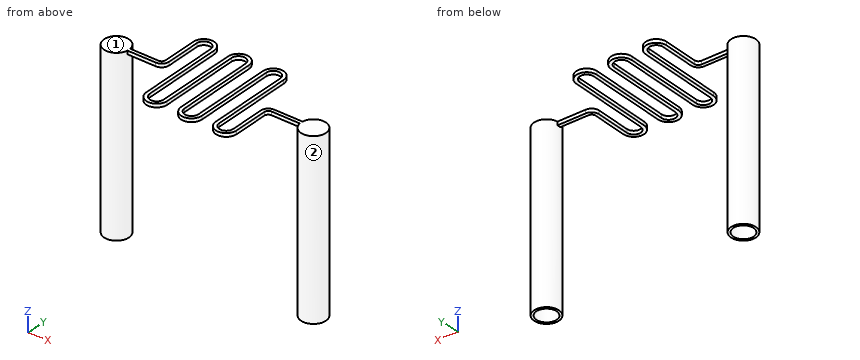
from build123d import *

# Parameters (mm, degrees)
BOSS_EXTRUDE1_DEPTH = 0.6
SKETCH3_W           = 2.15
SKETCH3_H           = 30
SKETCH4_W           = 2.15
SKETCH4_H           = 30
SKETCH5_R           = 1.75
CUT_EXTRUDE1_DEPTH  = 29


with BuildPart() as part:
    # Sketch2 → Boss-Extrude1 (new body)
    with BuildSketch(Plane.XY):
        with BuildLine():
            Line((-20.5, -0.3), (-13.5, -0.3))
            ThreePointArc((-13.5, -0.3), (-12.580761184, 0.080761184), (-12.2, 1))
            Line((-12.2, 1), (-12.2, 7))
            ThreePointArc((-12.2, 7), (-11, 8.2), (-9.8, 7))
            Line((-9.8, 7), (-9.8, 0))
            Line((-9.8, 0), (-9.8, -7))
            ThreePointArc((-9.8, -7), (-8, -8.8), (-6.2, -7))
            Line((-6.2, -7), (-6.2, 0))
            Line((-6.2, 0), (-6.2, 7))
            ThreePointArc((-6.2, 7), (-5, 8.2), (-3.8, 7))
            Line((-3.8, 7), (-3.8, 0))
            Line((-3.8, 0), (-3.8, -7))
            ThreePointArc((-3.8, -7), (-2, -8.8), (-0.2, -7))
            Line((-0.2, -7), (-0.2, 0))
            Line((-0.2, 0), (-0.2, 7))
            ThreePointArc((-0.2, 7), (1, 8.2), (2.2, 7))
            Line((2.2, 7), (2.2, 0))
            Line((2.2, 0), (2.2, -7))
            ThreePointArc((2.2, -7), (4, -8.8), (5.8, -7))
            Line((5.8, -7), (5.8, -1))
            ThreePointArc((5.8, -1), (6.005025253, -0.505025253), (6.5, -0.3))
            Line((6.5, -0.3), (13.5, -0.3))
            ThreePointArc((13.5, -0.3), (13.8, 0), (13.5, 0.3))
            Line((13.5, 0.3), (6.5, 0.3))
            ThreePointArc((6.5, 0.3), (5.580761184, -0.080761184), (5.2, -1))
            Line((5.2, -1), (5.2, -7))
            ThreePointArc((5.2, -7), (4, -8.2), (2.8, -7))
            Line((2.8, -7), (2.8, 0))
            Line((2.8, 0), (2.8, 7))
            ThreePointArc((2.8, 7), (1, 8.8), (-0.8, 7))
            Line((-0.8, 7), (-0.8, 0))
            Line((-0.8, 0), (-0.8, -7))
            ThreePointArc((-0.8, -7), (-2, -8.2), (-3.2, -7))
            Line((-3.2, -7), (-3.2, 0))
            Line((-3.2, 0), (-3.2, 7))
            ThreePointArc((-3.2, 7), (-5, 8.8), (-6.8, 7))
            Line((-6.8, 7), (-6.8, 0))
            Line((-6.8, 0), (-6.8, -7))
            ThreePointArc((-6.8, -7), (-8, -8.2), (-9.2, -7))
            Line((-9.2, -7), (-9.2, 0))
            Line((-9.2, 0), (-9.2, 7))
            ThreePointArc((-9.2, 7), (-11, 8.8), (-12.8, 7))
            Line((-12.8, 7), (-12.8, 1))
            ThreePointArc((-12.8, 1), (-13.005025253, 0.505025253), (-13.5, 0.3))
            Line((-13.5, 0.3), (-20.5, 0.3))
            ThreePointArc((-20.5, 0.3), (-20.8, 0), (-20.5, -0.3))
        make_face()
    extrude(amount=BOSS_EXTRUDE1_DEPTH)

    # Sketch3 → Revolve1 (revolve)
    with BuildSketch(Plane(origin=(0, 0, 0), x_dir=(1, 0, 0), z_dir=(0, 1, 0))):
        with Locations((-21.575, 14.4)):
            Rectangle(SKETCH3_W, SKETCH3_H)
    revolve(axis=Axis((-20.5, 0, -29.4), (0, 0, 1)))

    # Sketch4 → Revolve2 (revolve)
    with BuildSketch(Plane(origin=(0, 0, 0), x_dir=(1, 0, 0), z_dir=(0, 1, 0)), mode=Mode.PRIVATE) as revolve2_sk:
        with Locations((14.575, 14.4)):
            Rectangle(SKETCH4_W, SKETCH4_H)
    revolve(revolve2_sk.sketch.rotate(Axis((13.5, 0, -29.4), (0, 0, 1)), 180), axis=Axis((13.5, 0, -29.4), (0, 0, 1)))

    # Sketch5 → Cut-Extrude1 (cut)
    with BuildSketch(Plane(origin=(0, 0, -29.4), x_dir=(-1, 0, 0), z_dir=(0, 0, -1))):
        with Locations((20.5, 0)):
            Circle(SKETCH5_R)
        with Locations((-13.5, 0)):
            Circle(SKETCH5_R)
    extrude(amount=-CUT_EXTRUDE1_DEPTH, mode=Mode.SUBTRACT)


solid = part.part
Input: part model. Units: mm. Frame: model coordinates. Face numbers are marked on the shaded views. Give positions to 0.01 mm unless a question says otherwise; leave off trailing zeros. Loops run counter-clockwise (first coordinate to the right, second up) from the corner with the lowest first, then second, coordinate; pieces in that order, holes last. Notation, with made-up numbers: (43, 32.25) -> (85, 32.25) arc R28 cw to (85, 61.25) -> close; hole circle Ø3 at (4.5, 67.25). An arc over 180 degrees is marked (long way). Answer as a JSON object with one key per item and string values. Group by question number.
Item 1: Pull-direction query (X, two-part tool) for the marked faces 1 and 2; classes: released by +X, released by -X, zero draft, split by the parting line, or undercut.
Item 2: Pin query (flat end, axial travel): P1, Ø1.5, axis at x = -5.5, y = 6.5, coming from the -Z side; P2, Ø0.7, axis at y = 0.5, z = 0, coming from the -X side; P3, Ø0.7, axis at y = 3, z = 0, coming from the +X side. Return the tip coordinate at first contact, or that it passes through.
Item 3: Cut plane C-C, the plane x = 13.5. Return the cut outline in (y, z), and give its area (3 significant figures).
Item 4: Cut plane A-A, the plane z = -10. Return the cut outline in (x, y).
Item 5: Line query: probe 1 along Y at (x, z) = (-20.5, -12.25); probe 2 along X at (y, z) = (1.5, -25.75); probe 3 along Z at (x, y) = (2.5, -2.75). Output: solid intervals per line, ascending.
Item 6: Cut plane D-D, the plane x = -8. Return the cut outline in (y, z).
Item 7: Cut plane B-B, the plane y = -4.5. Return the cut outline in (x, z).
Checks:
{
 "1": {"face 1": "zero draft", "face 2": "undercut"},
 "2": {"P1": "stops at z = 0", "P2": "stops at x = -22.64", "P3": "stops at x = 2.8"},
 "3": {"outline": "(-2.15, -29.4) -> (-1.75, -29.4) -> (-1.75, -0.4) -> (1.75, -0.4) -> (1.75, -29.4) -> (2.15, -29.4) -> (2.15, 0.6) -> (-2.15, 0.6) -> close", "area": "27.5 mm²"},
 "4": {"outline": "circle Ø4.3 at (-20.5, 0); circle Ø4.3 at (13.5, 0); hole circle Ø3.5 at (-20.5, 0); hole circle Ø3.5 at (13.5, 0)"},
 "5": {"probe 1": "y = -2.15 to -1.75, 1.75 to 2.15", "probe 2": "x = -22.04 to -21.4, -19.6 to -18.96, 11.96 to 12.6, 14.4 to 15.04", "probe 3": "z = 0 to 0.6"},
 "6": {"outline": "(-8.8, 0) -> (-8.2, 0) -> (-8.2, 0.6) -> (-8.8, 0.6) -> close"},
 "7": {"outline": "(-9.8, 0) -> (-9.2, 0) -> (-9.2, 0.6) -> (-9.8, 0.6) -> close; (-6.8, 0) -> (-6.2, 0) -> (-6.2, 0.6) -> (-6.8, 0.6) -> close; (-3.8, 0) -> (-3.2, 0) -> (-3.2, 0.6) -> (-3.8, 0.6) -> close; (-0.8, 0) -> (-0.2, 0) -> (-0.2, 0.6) -> (-0.8, 0.6) -> close; (2.2, 0) -> (2.8, 0) -> (2.8, 0.6) -> (2.2, 0.6) -> close; (5.2, 0) -> (5.8, 0) -> (5.8, 0.6) -> (5.2, 0.6) -> close"}
}
